```python
from build123d import *

# Parameters (mm, degrees)
F0_R     = 1.5
F1_DEPTH = 6.2


with BuildPart() as f1:
    # F0 (on Front) → F1 (new body)
    with BuildSketch(Plane.XZ):
        Polygon((-185, -180.191748), (-180, -185), (-160, -185), (-158, -183), (-154, -179), (-148, -179), (-144, -183), (144, -183), (148, -179), (154, -179), (158, -183), (160, -185), (180, -185), (185, -180), (185, 180), (180, 185), (-180, 185), (-185, 180), align=None)
        with Locations((-165, -165)):
            Circle(F0_R, mode=Mode.SUBTRACT)
        with Locations((-175, -145)):
            Circle(F0_R, mode=Mode.SUBTRACT)
        with Locations((-155, -145)):
            Circle(F0_R, mode=Mode.SUBTRACT)
        with Locations((-135, -179)):
            Circle(F0_R, mode=Mode.SUBTRACT)
        with Locations((-180.083222, -117.008445)):
            Circle(F0_R, mode=Mode.SUBTRACT)
        with Locations((-137.048456, -117.034667)):
            Circle(F0_R, mode=Mode.SUBTRACT)
        with Locations((-45, -179)):
            Circle(F0_R, mode=Mode.SUBTRACT)
        with Locations((-181.26, -85)):
            Circle(F0_R, mode=Mode.SUBTRACT)
        with Locations((-133, -85)):
            Circle(F0_R, mode=Mode.SUBTRACT)
        with Locations((-180.048456, -23.034667)):
            Circle(F0_R, mode=Mode.SUBTRACT)
        with Locations((-181.26, -3.72)):
            Circle(F0_R, mode=Mode.SUBTRACT)
        with Locations((-137.048456, -23.034667)):
            Circle(F0_R, mode=Mode.SUBTRACT)
        with Locations((-133, -10.07)):
            Circle(F0_R, mode=Mode.SUBTRACT)
        with Locations((45, -179)):
            Circle(F0_R, mode=Mode.SUBTRACT)
        with Locations((135, -179)):
            Circle(F0_R, mode=Mode.SUBTRACT)
        with Locations((165, -165)):
            Circle(F0_R, mode=Mode.SUBTRACT)
        with Locations((155, -145)):
            Circle(F0_R, mode=Mode.SUBTRACT)
        with Locations((175, -145)):
            Circle(F0_R, mode=Mode.SUBTRACT)
        with BuildLine():
            ThreePointArc((-80, -165), (-85, -170), (-90, -165))
            Line((-90, -165), (-90, -150))
            Line((-90, -150), (-105, -135))
            Line((-105, -135), (-125, -135))
            Line((-125, -135), (-130, -130))
            Line((-130, -130), (-130, 140))
            Line((-130, 140), (-125, 145))
            Line((-125, 145), (125, 145))
            Line((125, 145), (130, 140))
            Line((130, 140), (130, -130))
            Line((130, -130), (125, -135))
            Line((125, -135), (105, -135))
            Line((105, -135), (90, -150))
            Line((90, -150), (90, -165))
            ThreePointArc((90, -165), (85, -170), (80, -165))
            Line((80, -165), (80, -150))
            Line((80, -150), (75, -145))
            Line((75, -145), (30, -145))
            Line((30, -145), (5, -170))
            Line((5, -170), (-5, -170))
            Line((-5, -170), (-30, -145))
            Line((-30, -145), (-75, -145))
            Line((-75, -145), (-80, -150))
            Line((-80, -150), (-80, -165))
        make_face(mode=Mode.SUBTRACT)
        with BuildLine():
            ThreePointArc((-179.162686, 85.675875), (-178.710798, 85.144061), (-178.548456, 84.465333))
            ThreePointArc((-178.548456, 84.465333), (-179.389216, 83.117964), (-180.968992, 83.281013))
            ThreePointArc((-180.968992, 83.281013), (-181.280779, 85.394803), (-179.162686, 85.675875))
        make_face(mode=Mode.SUBTRACT)
        with BuildLine():
            ThreePointArc((-136.162686, 85.675875), (-135.710798, 85.144061), (-135.548456, 84.465333))
            ThreePointArc((-135.548456, 84.465333), (-136.389216, 83.117964), (-137.968992, 83.281013))
            ThreePointArc((-137.968992, 83.281013), (-138.280779, 85.394803), (-136.162686, 85.675875))
        make_face(mode=Mode.SUBTRACT)
        with Locations((-175, 175)):
            Circle(F0_R, mode=Mode.SUBTRACT)
        with Locations((-155, 175)):
            Circle(F0_R, mode=Mode.SUBTRACT)
        with Locations((155, 175)):
            Circle(F0_R, mode=Mode.SUBTRACT)
        with Locations((175, 175)):
            Circle(F0_R, mode=Mode.SUBTRACT)
    extrude(amount=F1_DEPTH)


solid = f1.part
```
The model under review builds one solid part; all positions refer to its coordinate system, in mm. A direction names the side the tool comes from. Give positions to 0.01 mm unless a question says otherwise; leave off trailing zeros. Write each loop counter-clockwise with the first axis right and the second up, starting at its lowest first coordinate (ties: lowest second). Pieces come first, ordered by that corner, then holes. Notation, with made-up numbers: (87, 64.25) -> (127, 64.25) arc R29 cw to (127, 90.25) -> close; hole circle Ø4 at (-31, -28). An arc over 180 degrees is marked (long way). Answer in a Markdown table with one row per item.
1) Mouldability with a two-part tool opening along Z and no side actions: class faces 1 (the flat face through (98, -3, -142)), 2 (the flat face through (-3, -6.2, 167)) as +Z half, -Z half, draft (parallel to the pull), parting line (faces both ways), or undercut.
Worked answers:
| item | result |
|---|---|
| face 1 | undercut |
| face 2 | draft |
2) Clearance check with a flat-ended pin moving along its axis: P1, Ø1.8, axis at x = 155, z = 175, coming from the -Y side. State where the tip first meets the part, or that it passes through.
Worked answers:
| item | result |
|---|---|
| P1 | through |
3) Tool access review of faces 3 (the flat face through (-97, -3, -143)), 4 (the flat face through (-3, 0, 167)): name each direction out of +Z, -Z, +X, -X, +Y, -Y from which nothing blocks a thin tool from reaching the whole face with its end or side.
Worked answers:
| item | result |
|---|---|
| face 3 | +Y, -Y |
| face 4 | +Z, -Z, +X, -X, +Y |
4) For L1, parallel to Z at x = -175, y = -2.75; L2, parallel to X at y = -0.25, z = -57; L3, parallel to Z at x = -154.5, y = -1.5, list the stretches that pass through material, from the lowest coordinate up. Write a range as [from, to].
Worked answers:
| item | result |
|---|---|
| L1 | [-185, -146.5], [-143.5, 173.5], [176.5, 185] |
| L2 | [-185, -130], [130, 185] |
| L3 | [-179.5, -146.41], [-143.59, 173.59], [176.41, 185] |
5) Add section C-C on y = -3.5. Count the separate pieces of the cut face and the enclosed holes in it, plus the area to 3 significant figures.
Worked answers:
| item | result |
|---|---|
| separate pieces | 1 |
| enclosed holes | 25 |
| area | 59,800 mm² |
6) Add section B-B on z = -72.5. State the section outline as (x, y) points, plus the area to 3 significant figures.
Worked answers:
| item | result |
|---|---|
| outline | (-185, -6.2) -> (-130, -6.2) -> (-130, 0) -> (-185, 0) -> close; (130, -6.2) -> (185, -6.2) -> (185, 0) -> (130, 0) -> close |
| area | 682 mm² |
7) Add section A-A on x = 118. State the section outline as (y, z) points, plus the area to 3 significant figures.
Worked answers:
| item | result |
|---|---|
| outline | (-6.2, -183) -> (0, -183) -> (0, -135) -> (-6.2, -135) -> close; (-6.2, 145) -> (0, 145) -> (0, 185) -> (-6.2, 185) -> close |
| area | 546 mm² |
